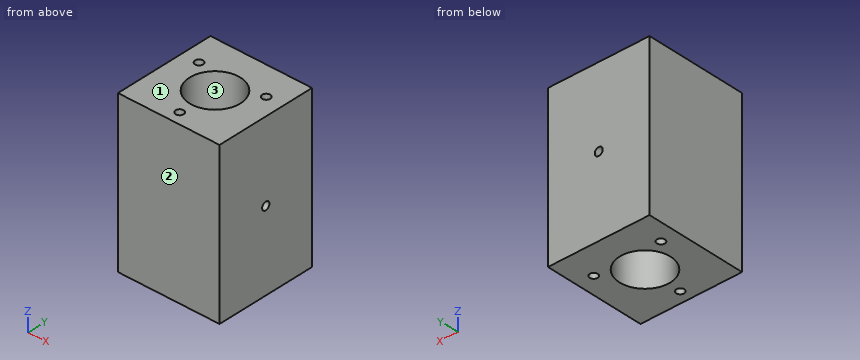
```python
from build123d import *

# Parameters (mm, degrees)
SKETCH1_W                  = 31.75
SKETCH1_H                  = 31.75
SKETCH1_R                  = 7.9375
SKETCH1_R_2                = 1.25
BOSS_EXTRUDE1_DEPTH        = 25
M3X0_5_TAPPED_HOLE1_REACH  = 45.417
M3X0_5_TAPPED_HOLE1_BORE_R = 1.25
M3X0_5_TAPPED_HOLE2_REACH  = 45.417
M3X0_5_TAPPED_HOLE2_BORE_R = 1.25


with BuildPart() as part:
    # Sketch1 → Boss-Extrude1 (new, symmetric)
    with BuildSketch(Plane.XY):
        Rectangle(SKETCH1_W, SKETCH1_H)
        Circle(SKETCH1_R, mode=Mode.SUBTRACT)
        with Locations((-10.5, 6.062177826)):
            Circle(SKETCH1_R_2, mode=Mode.SUBTRACT)
        with Locations((10.5, 6.062177826)):
            Circle(SKETCH1_R_2, mode=Mode.SUBTRACT)
        with Locations((0, -12.124355653)):
            Circle(SKETCH1_R_2, mode=Mode.SUBTRACT)
    extrude(amount=BOSS_EXTRUDE1_DEPTH, both=True)

    # M3x0.5 Tapped Hole1 bore → M3x0.5 Tapped Hole1 (cut, up to next)
    with BuildSketch(Plane(origin=(0, 15.875, 0), x_dir=(1, 0, 0), z_dir=(0, 1, 0)), mode=Mode.PRIVATE) as m3x0_5_tapped_hole1_sk1:
        Circle(M3X0_5_TAPPED_HOLE1_BORE_R)
    m3x0_5_tapped_hole1_tool1 = extrude(m3x0_5_tapped_hole1_sk1.sketch, amount=-M3X0_5_TAPPED_HOLE1_REACH, mode=Mode.PRIVATE) & part.part
    add(m3x0_5_tapped_hole1_tool1.solids().sort_by_distance((0, 15.875, 0))[0], mode=Mode.SUBTRACT)

    # M3x0.5 Tapped Hole2 bore → M3x0.5 Tapped Hole2 (cut, up to next)
    with BuildSketch(Plane(origin=(15.875, 0, 0), x_dir=(0, 0, -1), z_dir=(1, 0, 0)), mode=Mode.PRIVATE) as m3x0_5_tapped_hole2_sk1:
        Circle(M3X0_5_TAPPED_HOLE2_BORE_R)
    m3x0_5_tapped_hole2_tool1 = extrude(m3x0_5_tapped_hole2_sk1.sketch, amount=-M3X0_5_TAPPED_HOLE2_REACH, mode=Mode.PRIVATE) & part.part
    add(m3x0_5_tapped_hole2_tool1.solids().sort_by_distance((15.875, 0, 0))[0], mode=Mode.SUBTRACT)


solid = part.part
```
CAD build for the part. Positions are in the model's coordinates, mm. Face numbers are marked on the shaded views. Round coordinates to 2 decimals unless told otherwise and drop trailing zeros. Write each loop counter-clockwise with the first axis right and the second up, starting at its lowest first coordinate (ties: lowest second). Pieces come first, ordered by that corner, then holes. Notation, with made-up numbers: (86, -24.75) - (120, -24.75) arc R25 cw to (120, 11.25) - close; hole circle Ø9 at (16, 25.25). An arc over 180 degrees is marked (long way). Return JSON: item names as keys, results as strings. Group by question number.
Item 1: Band-saw the part on A-A on y = 0. State how many separate pieces and enclosed holes the cut face has, plus the area to 3 significant figures.
Item 2: Band-saw the part on C-C on x = -10.5. List the corners of the cut face in (y, z) (3 decimals), plus the area to 3 significant figures.
Item 3: Flat gauge pin, fed straight in: pin 1 Ø2 at (x, y) = (10.5, 6.06) entering from -Z. Where does the tip first touch, or does it go through?
Item 4: Mould opens along Y. For the marked faces 1, 2 and 3 say: +Y half, -Y half, draft (parallel to the pull), parting line (faces both ways), or undercut.
Item 5: Probe probe 1 along Y at (x, z) = (10.5, -3) (3 decimals); probe 2 along X at (y, z) = (-12, 10) (3 decimals); probe 3 along Y at (x, z) = (0, -12) (1 decimal). List the from-to ranges inside material, lowest first.
Item 6: Band-saw the part on B-B on x = 10.5. List the corners of the cut face in (y, z) (3 decimals).
Resolved:
{
 "1": {"separate pieces": "3", "enclosed holes": "0", "area": "774 mm²"},
 "2": {"outline": "(-15.875, -25) - (4.812, -25) - (4.812, 25) - (-15.875, 25) - close; (7.312, -25) - (15.875, -25) - (15.875, 25) - (7.312, 25) - close", "area": "1,460 mm²"},
 "3": {"pin 1": "passes through"},
 "4": {"face 1": "draft", "face 2": "-Y half", "face 3": "undercut"},
 "5": {"probe 1": "y = -15.875 to 4.812, 7.312 to 15.875", "probe 2": "x = -15.875 to -1.244, 1.244 to 15.875", "probe 3": "y = -15.9 to -13.4, -10.9 to -7.9, 7.9 to 15.9"},
 "6": {"outline": "(-15.875, -25) - (4.812, -25) - (4.812, 25) - (-15.875, 25) - close; (7.312, -25) - (15.875, -25) - (15.875, 25) - (7.312, 25) - close; hole circle Ø2.5 at (0, 0)"}
}
